The model under review builds one solid part; all positions refer to its coordinate system, in mm. A direction names the side the tool comes from. Coordinates: 2 decimals unless noted, no trailing zeros. Write each loop counter-clockwise with the first axis right and the second up, starting at its lowest first coordinate (ties: lowest second). Pieces come first, ordered by that corner, then holes. Notation, with made-up numbers: (45.5, 77.5) - (75.5, 77.5) arc R19 ccw to (75.5, 82.5) - close; hole circle Ø6 at (-18.5, -2.75). An arc over 180 degrees is marked (long way). Put each result on its own line as item: value.
from build123d import *

# Parameters (mm, degrees)
F0_R         = 11.3
F0_R_2       = 9
F1_DEPTH     = 15
F2_R         = 11.3
F3_DEPTH     = 2
F5_START     = -5
F4_R         = 9.5
F4_R_2       = 7.1437360255
F5_DEPTH     = 3.1
F7_W         = 50
F7_H         = 12
F8_DEPTH     = 2
F9_R         = 3
F10_W        = 1
F10_H        = 12
F10_W_2      = 12
F10_H_2      = 1
F11_DEPTH    = 10
F12_SIZE     = 1.2
F13_T2_ANGLE = 179.6107254138
F13_T4_ANGLE = 179.6107254138
F13_T6_ANGLE = 179.6107254138
F13_T8_ANGLE = 179.6107254138


# Not quite as in the source:
# - a fillet or chamfer that OpenCascade refuses, or shapes differently, is made with other operations: its cross-section is extruded or revolved along the edge and cut away or added


with BuildPart() as f1:
    # F0 (on Top) → F1 (new body)
    with BuildSketch(Plane.XY):
        Circle(F0_R)
        Circle(F0_R_2, mode=Mode.SUBTRACT)
    extrude(amount=F1_DEPTH)

    # F2 (on face) → F3 (join)
    with BuildSketch(Plane.XY.offset(15)):
        Circle(F2_R)
    extrude(amount=F3_DEPTH)

    # F4 (on face) → F5 (cut)
    with BuildSketch(Plane(origin=(0, 0, 0), x_dir=(1, 0, 0), z_dir=(0, 0, -1)).offset(F5_START)):
        Circle(F4_R)
        Circle(F4_R_2, mode=Mode.SUBTRACT)
    extrude(amount=-F5_DEPTH, mode=Mode.SUBTRACT)

    # F6: fillet of radius 1.5 on 3 edges, made by hand

    # F6_s1 → F6_t2 (revolve)
    with BuildSketch(Plane.XZ):
        with BuildLine():
            ThreePointArc((9, 5), (9.3693063938, 5.5056615531), (9.5, 6.1180339887))
            Line((9.5, 6.1180339887), (9.53, 6.1180339887))
            Line((9.53, 6.1180339887), (9.53, 5))
            Line((9.53, 5), (9.5, 4.97))
            ThreePointArc((9.5, 4.97), (9.25, 4.97), (9.02, 4.9776393202))
            Line((9.02, 4.9776393202), (9, 5))
        make_face()
    revolve(axis=Axis((0, 0, 5), (0, 0, -1)))

    # F6_s3 → F6_t4 (revolve)
    with BuildSketch(Plane.XZ):
        with BuildLine():
            ThreePointArc((9.5, 6.9819660113), (9.3693063938, 7.5943384469), (9, 8.1))
            Line((9, 8.1), (9.02, 8.1223606798))
            ThreePointArc((9.02, 8.1223606798), (9.25, 8.13), (9.5, 8.13))
            Line((9.5, 8.13), (9.53, 8.1))
            Line((9.53, 8.1), (9.53, 6.9819660113))
            Line((9.53, 6.9819660113), (9.5, 6.9819660113))
        make_face()
    revolve(axis=Axis((0, 0, 8.1), (0, 0, -1)))

    # F7 (on face) → F8 (join)
    with BuildSketch(Plane.XY.offset(17)):
        Rectangle(F7_W, F7_H)
    extrude(amount=-F8_DEPTH)

    # F9
    f9_edges = [f1.edges().sort_by_distance(p)[0] for p in [
        (-25, 6, 16),
        (-25, -6, 16),
        (25, 6, 16),
        (25, -6, 16),
    ]]
    fillet(f9_edges, radius=F9_R)

    # F10 (on face) → F11 (cut)
    with BuildSketch(Plane(origin=(0, 0, 0), x_dir=(1, 0, 0), z_dir=(0, 0, -1))):
        with Locations((0, -6.5)):
            Rectangle(F10_W, F10_H)
        with Locations((-6.5, 0)):
            Rectangle(F10_W_2, F10_H_2)
        Rectangle(F10_W, F10_H_2)
        with Locations((6.5, 0)):
            Rectangle(F10_W_2, F10_H_2)
        with Locations((0, 6.5)):
            Rectangle(F10_W, F10_H)
    extrude(amount=-F11_DEPTH, mode=Mode.SUBTRACT)

    # F12
    f12_edges = [f1.edges().sort_by_distance(p)[0] for p in [
        (6.363961, 6.363961, 0),
        (-6.363961, 6.363961, 0),
        (-6.363961, -6.363961, 0),
        (6.363961, -6.363961, 0),
    ]]
    chamfer(f12_edges, length=F12_SIZE)

    # F13: fillet of radius 8 on 4 edges, made by hand

    # F13_s1 → F13_t2 (revolve, cut)
    with BuildSketch(Plane(origin=(0, 0, 0), x_dir=(0, 0, 1), z_dir=(0.7095047819, -0.7047006205, 0))):
        with BuildLine():
            ThreePointArc((0, -10.2), (2.0233712711, -9.3058463753), (4.2142615011, -9))
            Line((4.2142615011, -9), (1.2, -9))
            Line((1.2, -9), (0, -10.2))
        make_face()
    revolve(axis=Axis((0, 0, 1.2), (0, 0, 1)), revolution_arc=F13_T2_ANGLE, mode=Mode.SUBTRACT)

    # F13_s3 → F13_t4 (revolve, cut)
    with BuildSketch(Plane(origin=(0, 0, 0), x_dir=(0, 0, 1), z_dir=(0.7047006205, 0.7095047819, 0))):
        with BuildLine():
            ThreePointArc((0, -10.2), (2.0233712711, -9.3058463753), (4.2142615011, -9))
            Line((4.2142615011, -9), (1.2, -9))
            Line((1.2, -9), (0, -10.2))
        make_face()
    revolve(axis=Axis((0, 0, 1.2), (0, 0, 1)), revolution_arc=F13_T4_ANGLE, mode=Mode.SUBTRACT)

    # F13_s5 → F13_t6 (revolve, cut)
    with BuildSketch(Plane(origin=(0, 0, 0), x_dir=(0, 0, 1), z_dir=(-0.7047006205, -0.7095047819, 0))):
        with BuildLine():
            ThreePointArc((0, -10.2), (2.0233712711, -9.3058463753), (4.2142615011, -9))
            Line((4.2142615011, -9), (1.2, -9))
            Line((1.2, -9), (0, -10.2))
        make_face()
    revolve(axis=Axis((0, 0, 1.2), (0, 0, 1)), revolution_arc=F13_T6_ANGLE, mode=Mode.SUBTRACT)

    # F13_s7 → F13_t8 (revolve, cut)
    with BuildSketch(Plane(origin=(0, 0, 0), x_dir=(0, 0, 1), z_dir=(-0.7095047819, 0.7047006205, 0))):
        with BuildLine():
            ThreePointArc((0, -10.2), (2.0233712711, -9.3058463753), (4.2142615011, -9))
            Line((4.2142615011, -9), (1.2, -9))
            Line((1.2, -9), (0, -10.2))
        make_face()
    revolve(axis=Axis((0, 0, 1.2), (0, 0, 1)), revolution_arc=F13_T8_ANGLE, mode=Mode.SUBTRACT)


solid = f1.part
1. To check wall thickness, follow probe 1 along X at (y, z) = (0, 10.5); probe 2 along Z at (x, y) = (-2, -8.25). State the ranges of each line that lie inside material, in increasing order.
Determined:
probe 1: x = -11.3 to -9, 9 to 11.3
probe 2: z = 15 to 17
2. Machinability: for faces 4 (the cylindrical face through (-6.43, -6.3, 4.6)), 5 (the flat face through (10, 0, 10)), 6 (the cylindrical face through (6.786, -6.648, 6.544)), 7 (the flat face through (0.5, -10, 5)), 8 (the flat face through (-25, 0, 16)), which of the approach directions +Z, -Z, +X, -X, +Y, -Y give a long, thin tool a straight path to every point of the face, cutting with its end or side? Answer none if there is none.
Determined:
face 4: -Z
face 5: -Z, +X, -X
face 6: none
face 7: -Z, +Y, -Y
face 8: +Z, -Z, -X, +Y, -Y
3. Consider section B-B on y = 0. State the section outline as (x, z) points, plus the area to 3 significant figures.
Determined:
outline: (-25, 15) - (-11.3, 15) - (-11.3, 10) - (-9, 10) - (-9, 15) - (9, 15) - (9, 10) - (11.3, 10) - (11.3, 15) - (25, 15) - (25, 17) - (-25, 17) - close
area: 123 mm^2
4. Consider section D-D on z = 12.5. State the section outline as (x, y) points.
Determined:
outline: circle Ø22.6 at (0, 0); hole circle Ø18 at (0, 0)
5. Consider section A-A on z = 8.75. State the section outline as (x, y) points.
Determined:
outline: (-11.29, -0.5) arc R11.3 ccw to (-0.5, -11.29) - (-0.5, -8.99) arc R9 cw to (-8.99, -0.5) - close; (-11.29, 0.5) - (-8.99, 0.5) arc R9 cw to (-0.5, 8.99) - (-0.5, 11.29) arc R11.3 ccw to start; (0.5, -11.29) arc R11.3 ccw to (11.29, -0.5) - (8.99, -0.5) arc R9 cw to (0.5, -8.99) - close; (0.5, 8.99) arc R9 cw to (8.99, 0.5) - (11.29, 0.5) arc R11.3 ccw to (0.5, 11.29) - close
6. For pin 1 Ø4 at (x, z) = (-6.5, 8) entering from -Y; pin 2 Ø10 at (y, z) = (9, 13) entering from +X; pin 3 Ø6 at (x, y) = (16, 0.5) entering from -Z, all flat-tipped, find the tip position at first contact; note any pin that passes through.
Determined:
pin 1: stops at y = -10.37
pin 2: stops at x = 24.64
pin 3: stops at z = 15
7. The part is to be moulded in two halves that separate along Y. For faces 1 (the cylindrical face through (10.78, 3.39, 8.38)), 2 (the flat face through (-10, 0, 10)), 3 (the flat face through (17, 0, 15)), say which applies: +Y half, -Y half, draft (parallel to the pull), parting line (faces both ways), or undercut.
Determined:
face 1: parting line
face 2: undercut
face 3: draft
8. Consider section C-C on x = 0. State the section outline as (y, z) points, plus the area to 3 significant figures.
Determined:
outline: (-11.3, 10) - (-9, 10) - (-9, 15) - (9, 15) - (9, 10) - (11.3, 10) - (11.3, 17) - (-11.3, 17) - close
area: 68.2 mm^2
